Autodesk Inventor part; units mm, degrees
ref_plane "YZ Plane" through (0, 0, 0) normal (1, 0, 0) x (0, 1, 0)
ref_plane "XZ Plane" through (0, 0, 0) normal (0, 1, 0) x (-1, 0, 0)
ref_plane "XY Plane" through (0, 0, 0) normal (0, 0, 1) x (1, 0, 0)
sketch "Sketch1" plane through (0, 0, 0) normal (0, 1, 0) x (-1, 0, 0)
  line L0 (210, 350) -> (-210, 350)
  line L1 (-210, 350) -> (-210, -350)
  line L2 (-210, -350) -> (210, -350)
  line L3 (210, -350) -> (210, 350)
  point P0 (0, 0)
  point P1 (210, 0)
  point P2 (0, -350)
  dimension "d0" = 420
  dimension "d1" = 700
extrude "Extrusion1" add sketch "Sketch1" along normal blind 15
sketch "Sketch2" plane through (0, 15, 0) normal (0, 1, 0) x (1, 0, 0)
  line L0 (-172.5, -279.5) -> (172.5, -279.5) construction
  line L1 (172.5, -279.5) -> (172.5, 169.5) construction
  line L2 (172.5, 169.5) -> (-172.5, 169.5) construction
  line L3 (-172.5, 169.5) -> (-172.5, -279.5) construction
  line L4 (-210, 350) -> (-210, -350) construction
  line L5 (210, 350) -> (-210, 350) construction
  line L6 (-210, -350) -> (210, -350) construction
  line L7 (-172.5, 144.5) -> (-172.5, 279.5) construction
  line L8 (-163.5, 144.5) -> (-163.5, 279.5)
  line L9 (-181.5, 279.5) -> (-181.5, 144.5)
  arc A0 (-181.5, 144.5) -> (-163.5, 144.5) centre (-172.5, 144.5) ccw
  arc A1 (-163.5, 279.5) -> (-181.5, 279.5) centre (-172.5, 279.5) ccw
  line L10 (-172.5, -169.5) -> (-172.5, -304.5) construction
  line L11 (-163.5, -169.5) -> (-163.5, -304.5)
  line L12 (-181.5, -304.5) -> (-181.5, -169.5)
  arc A2 (-163.5, -169.5) -> (-181.5, -169.5) centre (-172.5, -169.5) ccw
  arc A3 (-181.5, -304.5) -> (-163.5, -304.5) centre (-172.5, -304.5) ccw
  line L13 (172.5, -169.5) -> (172.5, -304.5) construction
  line L14 (181.5, -169.5) -> (181.5, -304.5)
  line L15 (163.5, -304.5) -> (163.5, -169.5)
  arc A4 (181.5, -169.5) -> (163.5, -169.5) centre (172.5, -169.5) ccw
  arc A5 (163.5, -304.5) -> (181.5, -304.5) centre (172.5, -304.5) ccw
  line L16 (172.5, 144.5) -> (172.5, 279.5) construction
  line L17 (181.5, 144.5) -> (181.5, 279.5)
  line L18 (163.5, 279.5) -> (163.5, 144.5)
  arc A6 (163.5, 144.5) -> (181.5, 144.5) centre (172.5, 144.5) ccw
  arc A7 (181.5, 279.5) -> (163.5, 279.5) centre (172.5, 279.5) ccw
  point P0 (0, 0)
  point P1 (0, 169.5)
  point P2 (-172.5, 212)
  point P3 (-172.5, -237)
  point P4 (172.5, -237)
  point P5 (172.5, 212)
  dimension "d5" = 180.5
  dimension "d7" = 18
  dimension "d9" = 25
  dimension "d10" = 110
  dimension "d11" = 110
  dimension "d12" = 25
  dimension "d46" = 345
  dimension "d47" = 449
extrude "Extrusion2" cut sketch "Sketch2" against normal blind 15
fillet "Fillet1" radius 30 2 edges at (-210, 7.5, 350) (-210, 7.5, -350)
sketch "Sketch3" plane through (0, 15, 0) normal (0, 1, 0) x (1, 0, 0)
  line L0 (147.5, -342.5) -> (192.5, -342.5) construction
  line L1 (147.5, -15.5) -> (192.5, -15.5) construction
  line L2 (147.5, 342.5) -> (192.5, 342.5) construction
  line L3 (-180, -350) -> (210, -350) construction
  line L4 (210, -350) -> (210, 350)
  point P0 (0, 0)
  dimension "d17" = 45
  dimension "d18" = 327
  dimension "d19" = 358
  dimension "d48" = 147.5
  dimension "d49" = 15.5
hole "Hole1" at (147.5, 15, 342.5) at (192.5, 15, 342.5) at (147.5, 15, 15.5) at (192.5, 15, 15.5) at (147.5, 15, -342.5) at (192.5, 15, -342.5) direction (0, -1, 0) diameter 9 end through all
sketch "Sketch4" plane through (0, 15, 0) normal (0, 1, 0) x (1, 0, 0)
  line L0 (210, 305) -> (140, 305)
  line L1 (140, 305) -> (140, 350)
  line L2 (210, 350) -> (-180, 350)
  line L3 (210, -350) -> (210, 350)
  point P0 (0, 0)
  point P1 (210, 285)
  dimension "d29" = 45
  dimension "d50" = 140
extrude "Extrusion3" cut sketch "Sketch4" against normal through all
sketch "Sketch5" plane through (0, 15, 0) normal (0, 1, 0) x (1, 0, 0)
  arc A0 (-163.5, -169.5) -> (-181.5, -169.5) centre (-172.5, -169.5) ccw
  line L0 (-163.5, -169.5) -> (-163.5, -304.5)
  arc A1 (-181.5, -304.5) -> (-163.5, -304.5) centre (-172.5, -304.5) ccw
  line L1 (-181.5, -304.5) -> (-181.5, -169.5)
  arc A2 (181.5, -169.5) -> (163.5, -169.5) centre (172.5, -169.5) ccw
  line L2 (181.5, -169.5) -> (181.5, -304.5)
  arc A3 (163.5, -304.5) -> (181.5, -304.5) centre (172.5, -304.5) ccw
  line L3 (163.5, -304.5) -> (163.5, -169.5)
  line L4 (-181.5, 144.5) -> (-181.5, 279.5)
  arc A4 (-163.5, 279.5) -> (-181.5, 279.5) centre (-172.5, 279.5) ccw
  line L5 (-163.5, 279.5) -> (-163.5, 144.5)
  arc A5 (-181.5, 144.5) -> (-163.5, 144.5) centre (-172.5, 144.5) ccw
  line L6 (163.5, 144.5) -> (163.5, 279.5)
  arc A6 (181.5, 279.5) -> (163.5, 279.5) centre (172.5, 279.5) ccw
  line L7 (181.5, 279.5) -> (181.5, 144.5)
  arc A7 (163.5, 144.5) -> (181.5, 144.5) centre (172.5, 144.5) ccw
  circle A8 centre (147.5, -342.5) radius 4.5
  circle A9 centre (192.5, -342.5) radius 4.5
  circle A10 centre (147.5, -15.5) radius 4.5
  circle A11 centre (192.5, -15.5) radius 4.5
  line L8 (140, 350) -> (-180, 350)
  arc A12 (-180, 350) -> (-210, 320) centre (-180, 320) ccw
  line L9 (-210, 320) -> (-210, -320)
  arc A13 (-210, -320) -> (-180, -350) centre (-180, -320) ccw
  line L10 (-180, -350) -> (210, -350)
  line L11 (210, -350) -> (210, 305)
  line L12 (210, 305) -> (140, 305)
  line L13 (140, 305) -> (140, 350)
  line L14 (-172.5, -304.5) -> (-172.5, -274.5) construction
  line L15 (-160, -304.5) -> (-160, -274.5)
  line L16 (-185, -274.5) -> (-185, -304.5)
  arc A14 (-185, -304.5) -> (-160, -304.5) centre (-172.5, -304.5) ccw
  arc A15 (-160, -274.5) -> (-185, -274.5) centre (-172.5, -274.5) ccw
  line L17 (172.5, -304.5) -> (172.5, -274.5) construction
  line L18 (185, -304.5) -> (185, -274.5)
  line L19 (160, -274.5) -> (160, -304.5)
  arc A16 (160, -304.5) -> (185, -304.5) centre (172.5, -304.5) ccw
  arc A17 (185, -274.5) -> (160, -274.5) centre (172.5, -274.5) ccw
  line L20 (172.5, 144.5) -> (172.5, 174.5) construction
  line L21 (185, 144.5) -> (185, 174.5)
  line L22 (160, 174.5) -> (160, 144.5)
  arc A18 (160, 144.5) -> (185, 144.5) centre (172.5, 144.5) ccw
  arc A19 (185, 174.5) -> (160, 174.5) centre (172.5, 174.5) ccw
  line L23 (-172.5, 144.5) -> (-172.5, 174.5) construction
  line L24 (-160, 144.5) -> (-160, 174.5)
  line L25 (-185, 174.5) -> (-185, 144.5)
  arc A20 (-185, 144.5) -> (-160, 144.5) centre (-172.5, 144.5) ccw
  arc A21 (-160, 174.5) -> (-185, 174.5) centre (-172.5, 174.5) ccw
  point P0 (0, 0)
  point P1 (-172.5, -289.5)
  point P2 (172.5, -289.5)
  point P3 (172.5, 159.5)
  point P4 (-172.5, 159.5)
  point P5 (163.5, -265.8253)
  point P6 (181.5, -265.8253)
  point P7 (163.5, 183.1747)
  point P8 (181.5, 183.1747)
  point P9 (-181.5, 183.1747)
  point P10 (-163.5, 183.1747)
  point P11 (-181.5, -265.8253)
  point P12 (-163.5, -265.8253)
  dimension "d35" = 25
  dimension "d36" = 30
  dimension "d37" = 30
  dimension "d38" = 30
  dimension "d39" = 30
  dimension "d40" = 25
  dimension "d41" = 25
  dimension "d42" = 25
extrude "Extrusion4" cut sketch "Sketch5" against normal through all contours A15 L15 A14 L16 L1 A1 L0 | A17 L18 A16 L19 L3 A3 L2 | A5 L5 A21 L24 A20 L25 L4 | A7 L7 A19 L21 A18 L22 L6
fillet "Fillet3" radius 10 8 edges at (163.5, 7.5, 265.8253) (181.5, 7.5, 265.8253) (163.5, 7.5, -183.1747) (181.5, 7.5, -183.1747) (-181.5, 7.5, -183.1747) (-163.5, 7.5, -183.1747) (-181.5, 7.5, 265.8253) (-163.5, 7.5, 265.8253)
equation "\"d0\" = width"
equation "\"d1\" = length"
equation "\"d7\" = slotdi"
equation "\"d9\" = slotb"
equation "\"d10\" = slota"
equation "\"d11\" = slota"
equation "\"d12\" = slotb"
equation "\"d35\" = slotaldi"
equation "\"d36\" = slotalign"
equation "\"d37\" = slotalign"
equation "\"d38\" = slotalign"
equation "\"d39\" = slotalign"
equation "\"d40\" = slotaldi"
equation "\"d41\" = slotaldi"
equation "\"d42\" = slotaldi"
equation "\"slota\" = 110"
equation "\"slotb\" = 25"
equation "\"slotdi\" = 18"
equation "\"slotalign\" = 30"
equation "\"slotaldi\" = 25"
equation "\"width\" = 420"
equation "\"length\" = 700"
properties part number "palp-desk" material "Aluminum 6061"
Read the model definition and answer for the solid it produces. Units are mm, in the model's axes. A direction names the side the tool comes from. Give positions to 0.01 mm unless a question says otherwise; leave off trailing zeros. Write each loop counter-clockwise with the first axis right and the second up, starting at its lowest first coordinate (ties: lowest second). Pieces come first, ordered by that corner, then holes. Notation, with made-up numbers: (-38, -12) - (-12, -12) arc R16 ccw to (-12, 11) - close; hole circle Ø1 at (-38.5, 21). An arc over 180 degrees is marked (long way). Return JSON: item names as keys, results as strings.
Q1. Given P1, Ø10.5, axis at x = 147.5, z = 15.5, coming from the +Y side, flat-ended and moving along its own axis, determine where the tip first touches the part or whether it passes through.
Reply:
{"P1": "y = 15"}
Q2. Consider line 1 along X through (y, z) = (3, 225); line 2 along Z through (x, y) = (172.5, 8.25); line 3 along Z through (x, y) = (192.5, 11.25). Determine where each line is inside the solid, lowest interval first. Write a range as [from, to].
Reply:
{"line 1": "[-210, -181.5], [-163.5, 163.5], [181.5, 210]", "line 2": "[-305, -288.5], [-132, 160.5], [317, 350]", "line 3": "[-305, 11], [20, 338], [347, 350]"}
Q3. A cutting plane is placed at A-A, the plane x = 172.5. Determine the outline of the cut face in (y, z), and give its area (3 significant figures).
Reply:
{"outline": "(0, -305) - (15, -305) - (15, -288.5) - (0, -288.5) - close; (0, -132) - (15, -132) - (15, 160.5) - (0, 160.5) - close; (0, 317) - (15, 317) - (15, 350) - (0, 350) - close", "area": "5,130 mm²"}
Q4. A cutting plane is placed at B-B, the plane z = -213. Determine the outline of the cut face in (x, y).
Reply:
{"outline": "(-210, 0) - (-181.5, 0) - (-181.5, 15) - (-210, 15) - close; (-163.5, 0) - (163.5, 0) - (163.5, 15) - (-163.5, 15) - close; (181.5, 0) - (210, 0) - (210, 15) - (181.5, 15) - close"}
Q5. For a pull along X with two mould halves and no side action, classify faces 1 (the face through (140, 8, -327)), 2 (the face through (172.698, 7.605, 160.502)), 3 (the face through (172.225, 7.605, -132.003)), 4 (the face through (-210, 7, -4)) as released by +X, released by -X, zero draft, split by the parting line, or undercut.
Reply:
{"face 1": "released by +X", "face 2": "undercut", "face 3": "undercut", "face 4": "released by -X"}
Q6. For faces 5 (the face through (12, 7, 350)), 6 (the face through (181.5, 8, 215)), determine the directions among +Z, -Z, +X, -X, +Y, -Y from which every point of the face is accessible in a straight line to the end or side of a thin tool.
Reply:
{"face 5": "+Z, +X, -X, +Y, -Y", "face 6": "+Y, -Y"}
Q7. A cutting plane is placed at C-C, the plane y = 3.25. Count the separate pieces of the cut face and the enclosed holes in it, and give its area (3 significant figures).
Reply:
{"separate pieces": "1", "enclosed holes": "8", "area": "278,000 mm²"}
